Read the model definition and answer for the solid it produces. Units are mm, in the model's axes. A direction names the side the tool comes from. Give positions to 0.01 mm unless a question says otherwise; leave off trailing zeros. Order: outer loops, then holes, each group sorted by start corner. A loop starts at its lowest first (then second) coordinate and runs counter-clockwise, first axis right, second up.
Item 1: Find the intervals of material crossed by line 1 along Y through (x, z) = (3.25, -12.5); line 2 along Z through (x, y) = (3.75, 7.5); line 3 along Z through (x, y) = (10.25, 5.75), in increasing order.
Item 2: Given pin 1 Ø1.4 at (x, z) = (5.5, -8) entering from +Y; pin 2 Ø2 at (x, z) = (6, -2.5) entering from +Y; pin 3 Ø3.5 at (x, z) = (9, -22.5) entering from +Y, each flat-ended and moving along its own axis, determine where each tip first touches the part or whether it passes through.
Item 3: A cutting plane is placed at B-B (z = -3.5). Write down the section's boundary in (x, y).
Item 4: A cutting plane is placed at A-A (x = 6.5). Write down the section's boundary in (y, z) (3 decimals).
Item 5: A cutting plane is placed at C-C (y = 4.75). Write down the section's boundary in (x, z), plus the area to 3 significant figures.
Item 6: A cutting plane is placed at D-D (x = 11.25). Write down the section's boundary in (y, z) (3 decimals).
Item 7: Which of the six approach directions +Z, -Z, +X, -X, +Y, -Y give full straight-line access (tool end or side, diameter ignored) to faces 1 (the face through (6.4, 2.1, -15.7)), 2 (the face through (6.4, 1, -24.7)), 3 (the face through (6, 4, -7))?
from build123d import *

# Parameters (mm, degrees)
SKETCH1_W                                      = 13
SKETCH1_H                                      = 25
BOSS_EXTRUDE1_DEPTH                            = 1
SKETCH3_W                                      = 13
SKETCH3_H                                      = 11
BOSS_EXTRUDE2_DEPTH                            = 7
SKETCH4_R                                      = 4.5
BOSS_EXTRUDE3_DEPTH                            = 13
SKETCH6_R                                      = 4
CUT_EXTRUDE1_DEPTH                             = 30.58042089
FILLET1_R                                      = 3
CSK_FOR_M3_OVAL_HEAD_MACHINE_SCREW2_AT_2_COUNT = 2
CSK_FOR_M3_OVAL_HEAD_MACHINE_SCREW2_AT_2_PITCH = 18


with BuildPart() as part:
    # Sketch1 → Boss-Extrude1 (new body)
    with BuildSketch(Plane(origin=(0, 0, 0), x_dir=(1, 0, 0), z_dir=(0, 1, 0))):
        with Locations((6.5, 12.5)):
            Rectangle(SKETCH1_W, SKETCH1_H)
    extrude(amount=BOSS_EXTRUDE1_DEPTH)

    # Sketch3 → Boss-Extrude2 (add)
    with BuildSketch(Plane(origin=(0, 1, 0), x_dir=(1, 0, 0), z_dir=(0, 1, 0))):
        with Locations((6.5, 12.5)):
            Rectangle(SKETCH3_W, SKETCH3_H)
    extrude(amount=BOSS_EXTRUDE2_DEPTH)

    # Sketch4 → Boss-Extrude3 (add, through all)
    with BuildSketch(Plane(origin=(13, 0, 0), x_dir=(0, 0, -1), z_dir=(1, 0, 0))):
        with Locations((12.5, 4.5)):
            Circle(SKETCH4_R)
    extrude(amount=-BOSS_EXTRUDE3_DEPTH)

    # Sketch6 → Cut-Extrude1 (cut, through all)
    with BuildSketch(Plane.ZY.offset(5e-05)):
        with Locations((-12.5, 4.5)):
            Circle(SKETCH6_R)
    extrude(amount=-CUT_EXTRUDE1_DEPTH, mode=Mode.SUBTRACT)

    # Fillet1
    fillet1_edges = [part.edges().sort_by_distance(p)[0] for p in [
        (6.5, 8, -15.328427125),
        (6.5, 8, -9.671572875),
    ]]
    fillet(fillet1_edges, radius=FILLET1_R)

    # Sketch15 → CSK for M3 Oval Head Machine Screw2 (revolve, cut)
    with BuildSketch(Plane(origin=(6.5, 1, -3.5), x_dir=(0, 0, 1), z_dir=(1, 0, 0))):
        Polygon((0, 0), (0, 1), (1.75, 1), (1.75, 1.25), (3, 0), align=None)
    csk_for_m3_oval_head_machine_screw2 = revolve(axis=Axis((6.5, 7.35, -3.5), (0, -1, 0)), mode=Mode.SUBTRACT)

    # CSK for M3 Oval Head Machine Screw2 at 2: CSK for M3 Oval Head Machine Screw2 ×2
    with Locations(*[(0, 0, -i * CSK_FOR_M3_OVAL_HEAD_MACHINE_SCREW2_AT_2_PITCH) for i in range(1, CSK_FOR_M3_OVAL_HEAD_MACHINE_SCREW2_AT_2_COUNT)]):
        add(csk_for_m3_oval_head_machine_screw2, mode=Mode.SUBTRACT)


solid = part.part
Response values:
1. line 1: y = 0 to 0.5, 8.5 to 9
1. line 2: z = -18 to -15.15, -9.85 to -7
1. line 3: z = -18 to -16.3, -8.7 to -7
2. pin 1: stops at y = 8
2. pin 2: stops at y = 0.12
2. pin 3: stops at y = 1
3. outline: (0, 0) - (4.5, 0) - (3.5, 1) - (0, 1) - close; (8.5, 0) - (13, 0) - (13, 1) - (9.5, 1) - close
4. outline: (0, -25) - (1, -25) - (1, -24.5) - (0, -23.5) - close; (0, -19.5) - (1, -18.5) - (1, -18) - (8, -18) - (8, -16.242) arc R3 cw to (8.4, -14.745) arc R4.5 ccw to (8.4, -10.255) arc R3 cw to (8, -8.758) - (8, -7) - (1, -7) - (1, -6.5) - (0, -5.5) - close; (0, -1.5) - (1, -0.5) - (1, 0) - (0, 0) - close; hole circle Ø8 at (4.5, -12.5)
5. outline: (0, -18) - (13, -18) - (13, -16.49) - (0, -16.49) - close; (0, -8.51) - (13, -8.51) - (13, -7) - (0, -7) - close
5. area: 39.2 mm2
6. outline: (0, -25) - (1, -25) - (1, -18) - (8, -18) - (8, -16.242) arc R3 cw to (8.4, -14.745) arc R4.5 ccw to (8.4, -10.255) arc R3 cw to (8, -8.758) - (8, -7) - (1, -7) - (1, 0) - (0, 0) - close; hole circle Ø8 at (4.5, -12.5)
7. face 1: +X, -X
7. face 2: -Z, +X, -X, +Y
7. face 3: +Z, +X, -X, +Y
